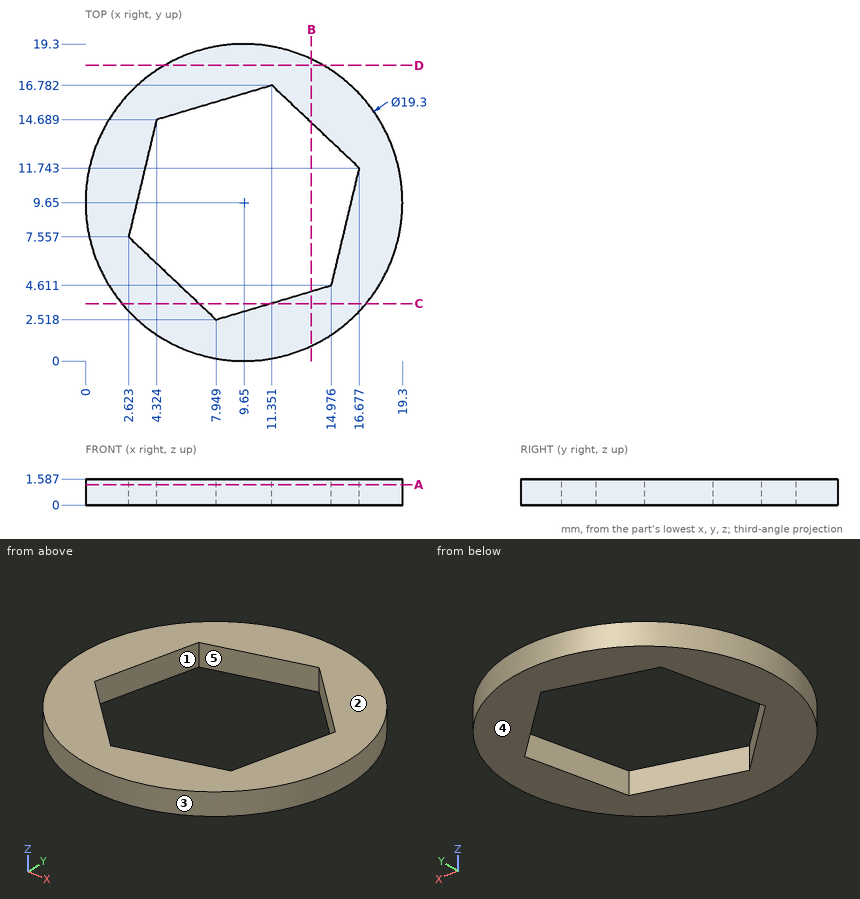
Drawing for the job (mm, zero at the part's lowest x, y, z). A direction names the side the tool comes from. Coordinates: 2 decimals unless noted, no trailing zeros. Write each loop counter-clockwise with the first axis right and the second up, starting at its lowest first coordinate (ties: lowest second). Pieces come first, ordered by that corner, then holes. Notation, with made-up numbers: (34, 33.25) -> (90, 33.25) arc R17 ccw to (90, 50.25) -> close; hole circle Ø6 at (54, 86.5). An arc over 180 degrees is marked (long way). One line per item, written item: value. Start each with the question number.
1) Slice it at D-D on y = 18. Write the cut outline in (x, z).
2) Slice it at B-B on x = 13.75. Write the cut outline in (y, z) (1 decimal).
3) Slice it at A-A on z = 1.25. Write the cut outline in (x, y).
4) Pull direction Y, two halves, no side cores. Call the marked faces 3, 4 and 5: +Y half, -Y half, draft (parallel to the pull), parting line (faces both ways), or undercut.
5) Slice it at C-C on y = 3.5. Write the cut outline in (x, z).
6) Probe probe 1 along Y at (x, z) = (5, 0.3) (1 decimal); probe 2 along X at (y, z) = (9.75, 0.95) (1 decimal); probe 3 along Y at (x, z) = (8, 1.3) (1 decimal). List the from-to ranges inside material, lowest first.
7) Which spindle directions (+Z, -Z, +X, -X, +Y, -Y) get a long thin tool onto all of the face, cutting with end or side? Do the marked faces 1 and 2. Say none if no direction does.
Answers follow:
1. outline: (4.81, 0) -> (14.49, 0) -> (14.49, 1.59) -> (4.81, 1.59) -> close
2. outline: (0.9, 0) -> (4.2, 0) -> (4.2, 1.6) -> (0.9, 1.6) -> close; (14.5, 0) -> (18.4, 0) -> (18.4, 1.6) -> (14.5, 1.6) -> close
3. outline: circle Ø19.3 at (9.65, 9.65); hole (2.62, 7.56) -> (7.95, 2.52) -> (14.98, 4.61) -> (16.68, 11.74) -> (11.35, 16.78) -> (4.32, 14.69) -> close
4. face 3: parting line
4. face 4: draft
4. face 5: undercut
5. outline: (2.21, 0) -> (6.91, 0) -> (6.91, 1.59) -> (2.21, 1.59) -> close; (11.25, 0) -> (17.09, 0) -> (17.09, 1.59) -> (11.25, 1.59) -> close
6. probe 1: 1.2 to 5.3, 14.9 to 18.1
6. probe 2: 0 to 3.1, 16.2 to 19.3
6. probe 3: 0.1 to 2.5, 15.8 to 19.2
7. face 1: +Z, -Z
7. face 2: +Z, +X, -X, +Y, -Y
